Geometry: final body of the model. Coordinates: model frame, mm. A direction names the side the tool comes from. Round coordinates to 2 decimals unless told otherwise and drop trailing zeros. Order: outer loops, then holes, each group sorted by start corner. A loop starts at its lowest first (then second) coordinate and runs counter-clockwise, first axis right, second up. Notation, with made-up numbers: (28, 15) -> (53, 15) arc R11 ccw to (53, 20) -> close; hole circle Ø3 at (42.25, 19.5). An arc over 180 degrees is marked (long way). Put each result on its own line as item: value.
```python
from build123d import *

# Parameters (mm, degrees)
F0_R     = 1.35
F1_DEPTH = 2.5
F0_W     = 3
F0_H     = 70
F2_DEPTH = 10
F3_R     = 1.35
F4_DEPTH = 3.001


with BuildPart() as f1:
    # F0 (on Top) → F1 (new body)
    with BuildSketch(Plane.XY):
        Polygon((19.589888, 61.650399), (19.589888, 71.650399), (-10.410112, 71.650399), (-10.410112, 61.650399), (-10.410112, -8.349601), (-0.410112, -8.349601), (-0.410112, 61.650399), align=None)
        with Locations((-5.410112, 66.650399)):
            Circle(F0_R, mode=Mode.SUBTRACT)
        with Locations((14.589888, 66.650399)):
            Circle(F0_R, mode=Mode.SUBTRACT)
    extrude(amount=F1_DEPTH)

    # F0 (on Top) → F2 (join)
    with BuildSketch(Plane.XY):
        with Locations((-11.910112, 26.650399)):
            Rectangle(F0_W, F0_H)
    extrude(amount=F2_DEPTH)

    # F3 (on face) → F4 (cut, through all)
    with BuildSketch(Plane.YZ.offset(-10.410112)):
        with Locations((-5.849601, 7.5)):
            Circle(F3_R)
        with Locations((59.150399, 7.5)):
            Circle(F3_R)
    extrude(amount=-F4_DEPTH, mode=Mode.SUBTRACT)


solid = f1.part
```
1. Cut plane B-B on x = 15. Return loops of the section in (y, z), and give its area (3 significant figures).
Ans:
outline: (61.65, 0) -> (65.36, 0) -> (65.36, 2.5) -> (61.65, 2.5) -> close; (67.94, 0) -> (71.65, 0) -> (71.65, 2.5) -> (67.94, 2.5) -> close
area: 18.6 mm²
2. Set-up query: faces 1 (the face through (9, 61.65, 1)), 2 (the face through (-2, 41, 2.5)), 3 (the face through (-11.889, 60.438, 7.906)), 4 (the face through (-12, 61.65, 5)), 5 (the face through (15.21, 65.45, 1.23)). Return all of +Z, -Z, +X, -X, +Y, -Y with unobstructed straight access to the full face (end or side cutting, diameter ignored); none if empty.
Ans:
face 1: +Z, -Z, +X, -Y
face 2: +Z, +X, +Y, -Y
face 3: +X, -X
face 4: +Z, -Z, -X, +Y
face 5: +Z, -Z
3. Cut plane D-D on z = 1. Return loops of the section in (x, y).
Ans:
outline: (-13.41, -8.35) -> (-0.41, -8.35) -> (-0.41, 61.65) -> (19.59, 61.65) -> (19.59, 71.65) -> (-10.41, 71.65) -> (-10.41, 61.65) -> (-13.41, 61.65) -> close; hole circle Ø2.7 at (-5.41, 66.65); hole circle Ø2.7 at (14.59, 66.65)
4. Cut plane C-C on y = 14.5. Return loops of the section in (x, z), and give its area (3 significant figures).
Ans:
outline: (-13.41, 0) -> (-0.41, 0) -> (-0.41, 2.5) -> (-10.41, 2.5) -> (-10.41, 10) -> (-13.41, 10) -> close
area: 55.0 mm²
5. Contact query for flat-ended pins moving along their axis: P1, Ø5, axis at x = 13.5, z = 1, coming from the -Y side; P2, Ø8, axis at x = -8.5, y = 16.5, coming from the +Z side; P3, Ø4, axis at y = 17.5, z = 7.5, coming from the +X side; P4, Ø4.5, axis at x = -5.41, y = 66.65, coming from the +Z side. Output: stop coordinate, or through.
Ans:
P1: y = 61.65
P2: z = 10
P3: x = -10.41
P4: z = 2.5
6. Material intervals for probe 1 along Z at (x, y) = (-4.5, 19.5); probe 2 along X at (y, z) = (52.5, 2); probe 3 along X at (y, z) = (38, 6.25), sorted ascending.
Ans:
probe 1: 0 to 2.5
probe 2: -13.41 to -0.41
probe 3: -13.41 to -10.41
7. Cut plane A-A on z = 7.5. Return loops of the section in (x, y).
Ans:
outline: (-13.41, -8.35) -> (-10.41, -8.35) -> (-10.41, -7.2) -> (-13.41, -7.2) -> close; (-13.41, -4.5) -> (-10.41, -4.5) -> (-10.41, 57.8) -> (-13.41, 57.8) -> close; (-13.41, 60.5) -> (-10.41, 60.5) -> (-10.41, 61.65) -> (-13.41, 61.65) -> close
8. Draft query along X for faces 6 (the face through (-4.79, 65.45, 1.23)), 7 (the face through (5, 71.65, 1)), 8 (the face through (-10.41, 67, 1)). Return one class per face: +X half, -X half, draft (parallel to the pull), parting line (faces both ways), or undercut.
Ans:
face 6: undercut
face 7: draft
face 8: -X half
